```python
from build123d import *

# Parameters (mm, degrees)
SKETCH1_W           = 15.875
SKETCH1_H           = 125.984
SKETCH1_W_2         = 1.905
SKETCH1_H_2         = 115.824
BOSS_EXTRUDE1_DEPTH = 4.064
SKETCH2_W           = 7.112
SKETCH2_H           = 115.824
CUT_EXTRUDE1_DEPTH  = 2.54
FILLET1_R           = 0.508
BOSS_EXTRUDE2_START = -4.064
SKETCH3_W           = 23.9522
SKETCH3_H           = 21.336
BOSS_EXTRUDE2_DEPTH = 4.064
SKETCH4_W           = 16.256
SKETCH4_H           = 16.256
CUT_EXTRUDE2_DEPTH  = 2.667
SKETCH5_W           = 18.796
SKETCH5_H           = 18.796
CUT_EXTRUDE3_DEPTH  = 1.016
SKETCH6_R           = 5.715
CUT_EXTRUDE4_DEPTH  = 2.54
CUT_EXTRUDE4_DRAFT  = -45
CHAMFER1_SIZE       = 8.128
CHAMFER1_SIZE_2     = 5.691286871
FILLET3_R           = 3.175
FILLET4_R           = 0.508
SKETCH7_W           = 2.286
SKETCH7_H           = 113.284
CUT_EXTRUDE5_DEPTH  = 128.045267433
BOSS_EXTRUDE3_DEPTH = 6.35
BOSS_EXTRUDE4_DEPTH = 6.35
SKETCH10_R          = 1.397
CUT_EXTRUDE6_DEPTH  = 129.316594879


with BuildPart() as part:
    # Sketch1 → Boss-Extrude1 (new body)
    with BuildSketch(Plane.XY):
        with Locations((7.9375, 62.992)):
            Rectangle(SKETCH1_W, SKETCH1_H)
        with Locations((9.5885, 62.992)):
            Rectangle(SKETCH1_W_2, SKETCH1_H_2, mode=Mode.SUBTRACT)
    extrude(amount=BOSS_EXTRUDE1_DEPTH)

    # Sketch2 → Cut-Extrude1 (cut)
    with BuildSketch(Plane.XY.offset(4.064)):
        with Locations((5.08, 62.992)):
            Rectangle(SKETCH2_W, SKETCH2_H)
    extrude(amount=-CUT_EXTRUDE1_DEPTH, mode=Mode.SUBTRACT)

    # Fillet1
    fillet1_edges = [part.edges().sort_by_distance(p)[0] for p in [
        (8.636, 62.992, 1.524),
    ]]
    fillet(fillet1_edges, radius=FILLET1_R)

    # Sketch3 → Boss-Extrude2 (add)
    with BuildSketch(Plane(origin=(0, 0, 0), x_dir=(-1, 0, 0), z_dir=(0, 0, -1)).offset(BOSS_EXTRUDE2_START)):
        with Locations((-3.8989, 115.316)):
            Rectangle(SKETCH3_W, SKETCH3_H)
    extrude(amount=BOSS_EXTRUDE2_DEPTH)

    # Sketch4 → Cut-Extrude2 (cut)
    with BuildSketch(Plane.XY.offset(4.064)):
        with Locations((2.5908, 115.316)):
            Rectangle(SKETCH4_W, SKETCH4_H)
    extrude(amount=-CUT_EXTRUDE2_DEPTH, mode=Mode.SUBTRACT)

    # Sketch5 → Cut-Extrude3 (cut)
    with BuildSketch(Plane.XY.offset(4.064)):
        with Locations((2.5908, 115.316)):
            Rectangle(SKETCH5_W, SKETCH5_H)
    extrude(amount=-CUT_EXTRUDE3_DEPTH, mode=Mode.SUBTRACT)


with BuildPart() as cut_extrude4_tool:
    # Sketch6 → Cut-Extrude4 (with draft: the straight prism first)
    with BuildSketch(Plane.XY.offset(1.397)):
        with Locations((2.5908, 115.316)):
            Circle(SKETCH6_R)
    extrude(amount=-CUT_EXTRUDE4_DEPTH)
    # Cut-Extrude4: the draft: its side faces are tilted about the plane it starts from
    cut_extrude4_sides = [cut_extrude4_tool.faces().sort_by_distance(p)[0] for p in [
        (-3.1242, 115.316, 0.127),
    ]]
    draft(cut_extrude4_sides, Plane.XY.offset(1.397), CUT_EXTRUDE4_DRAFT)


with BuildPart() as part_1:
    add(part.part)

    # Cut-Extrude4: cut by cut_extrude4_tool
    add(cut_extrude4_tool.part, mode=Mode.SUBTRACT)

    # Chamfer1
    # the kernel refuses this chamfer: 8.128, 5.691286871 mm, written as the material it adds along each edge
    with BuildSketch(Plane(origin=(0, 104.648, 4.064), x_dir=(-0.9997533347641298, 0.022209674198457242, 0), z_dir=(0, 0, -1))) as chamfer1_piece_1_section:
        Polygon((CHAMFER1_SIZE * 0.999753334764, -CHAMFER1_SIZE * 0.0222096741985), (-CHAMFER1_SIZE_2 * 0.0222096741968, -CHAMFER1_SIZE_2 * 0.999753334688), (0, 0), align=None)
    chamfer1_piece_1 = extrude(amount=4.064, mode=Mode.PRIVATE)
    chamfer1_piece_1 = split(chamfer1_piece_1, bisect_by=Plane(origin=(-8.0772, 102.794358519, 2.032), z_dir=(1, 0, 0)), keep=Keep.TOP, mode=Mode.PRIVATE)
    add(chamfer1_piece_1)

    # Fillet3
    fillet3_edges = [part_1.edges().sort_by_distance(p)[0] for p in [
        (0, 98.956713129, 2.032),
        (-8.0772, 104.612429457, 2.032),
        (-8.0772, 125.984, 2.032),
        (0, 0, 2.032),
    ]]
    fillet(fillet3_edges, radius=FILLET3_R)

    # Fillet4
    fillet4_edges = [part_1.edges().sort_by_distance(p)[0] for p in [
        (-3.1242, 115.316, 1.397),
    ]]
    fillet(fillet4_edges, radius=FILLET4_R)

    # Sketch7 → Cut-Extrude5 (cut, through all)
    with BuildSketch(Plane(origin=(0, 0, 0), x_dir=(-1, 0, 0), z_dir=(0, 0, -1))):
        with Locations((-14.732, 62.992)):
            Rectangle(SKETCH7_W, SKETCH7_H)
    extrude(amount=-CUT_EXTRUDE5_DEPTH, mode=Mode.SUBTRACT)

    # Sketch8 → Boss-Extrude3 (add)
    with BuildSketch(Plane(origin=(0, 125.984, 0), x_dir=(1, 0, 0), z_dir=(0, 1, 0))):
        with BuildLine():
            Line((15.875, 0), (17.653, 0))
            ThreePointArc((17.653, 0), (21.020596045, -8.130096045), (12.8905, -4.7625))
            Line((12.8905, -4.7625), (12.8905, -4.064))
            Line((12.8905, -4.064), (15.875, -4.064))
            Line((15.875, -4.064), (15.875, 0))
        make_face()
    extrude(amount=-BOSS_EXTRUDE3_DEPTH)

    # Sketch9 → Boss-Extrude4 (add)
    with BuildSketch(Plane(origin=(0, 6.35, 0), x_dir=(1, 0, 0), z_dir=(0, 1, 0))):
        with BuildLine():
            Line((17.653, 0), (13.589, 0))
            Line((13.589, 0), (13.589, -4.064))
            Line((13.589, -4.064), (12.8905, -4.064))
            Line((12.8905, -4.064), (12.8905, -4.7625))
            ThreePointArc((12.8905, -4.7625), (21.020596045, -8.130096045), (17.653, 0))
        make_face()
    extrude(amount=-BOSS_EXTRUDE4_DEPTH)

    # Sketch10 → Cut-Extrude6 (cut, through all)
    with BuildSketch(Plane(origin=(0, 125.984, 0), x_dir=(1, 0, 0), z_dir=(0, 1, 0))):
        with Locations(Location((17.653, -4.7625, 0), (0, 0, 270))):
            Circle(SKETCH10_R)
    extrude(amount=-CUT_EXTRUDE6_DEPTH, mode=Mode.SUBTRACT)


solid = part_1.part
```
Can you work these out from the model? Positions are in its coordinate system, mm. A direction names the side the tool comes from. Give positions to 0.01 mm unless a question says otherwise; leave off trailing zeros. Loops run counter-clockwise (first coordinate to the right, second up) from the corner with the lowest first, then second, coordinate; pieces in that order, holes last. Notation, with made-up numbers: M 19,82.25 L 66,82.25 A16 ccw 66,87.25 Z; hole C 46,87.5 d7. An arc over 180 degrees is marked long. Use CSV: the item, a comma, the result in double quotes. Start each with the question number.
1. Imagine slicing it at A-A, the plane y = 59.5. Write out the boundary of the cut face in (x, z).
2. For P1, Ø0.8, axis at y = 114, z = 3.5, coming from the +X side; P2, Ø3.5, axis at x = 5.5, y = 72, coming from the +Z side; P3, Ø8, axis at x = -1, y = 111.5, coming from the +Z side; P4, Ø3, axis at x = 9, y = 77.5, coming from the -Z side, each with a flat end and sliding along its axis, tell me the tip position at first contact or that it passes through.
3. If we mould it in two halves opening along Y, with no side actions, what happens to faces 1 (the face through (16.29, 3.22, 4.46)), 2 (the face through (1.524, 54, 3)), 3 (the face through (5, 56, 1.524)), 4 (the face through (-0.37, 98.79, 2))? For each: released by +Y, released by -Y, zero draft, split by the parting line, or undercut.
4. Imagine slicing it at B-B, the plane y = 102.5. Write out the boundary of the cut face in (x, z), plus the area to 3 significant figures.
5. On a 3-axis mill with a long thin cutter (end or side, diameter ignored), from which of +Z, -Z, +X, -X, +Y, -Y can I reach the whole of each face in a straight line? I mean faces 5 (the face through (15, 0, 4)), 6 (the face through (21.13, 122.853, 8.017)), 7 (the face through (0, 50, 2)), 8 (the face through (2, 124, 3.048)), 9 (the face through (10.541, 54, 2)). Say none if no direction works.
6. If I drill on L1, parallel to X at y = 56, z = 3.75; L2, parallel to Y at x = 17, z = 2; L3, parallel to X at y = 61, z = 1.25, over which ranges is the centre line in solid material (lowest first)?
Response values:
1,outline,"M 0,0 L 8.64,0 L 8.64,1.02 A0.51 ccw 8.13,1.52 L 1.52,1.52 L 1.52,4.06 L 0,4.06 Z; M 10.54,0 L 13.59,0 L 13.59,4.06 L 10.54,4.06 Z"
2,P1,"x = 13.59"
2,P2,"z = 1.52"
2,P3,"z = 1.4"
2,P4,"z = 0"
3,face 1,"zero draft"
3,face 2,"undercut"
3,face 3,"undercut"
3,face 4,"released by -Y"
4,outline,"M -5.06,0 L 8.64,0 L 8.64,1.02 A0.51 ccw 8.13,1.52 L 1.52,1.52 L 1.52,4.06 L -5.06,4.06 Z; M 10.54,0 L 13.59,0 L 13.59,4.06 L 10.54,4.06 Z"
4,area,"49.9 mm^2"
5,face 5,"+Z, -Z, +X, -X, -Y"
5,face 6,"+Y, -Y"
5,face 7,"+Z, -Z, -X, -Y"
5,face 8,"+Z"
5,face 9,"+Z, -Z"
6,L1,"0 to 1.52, 10.54 to 13.59"
6,L2,"0 to 6.35, 119.63 to 125.98"
6,L3,"0 to 8.58, 10.54 to 13.59"
